```python
from build123d import *

# Parameters (mm, degrees)
SKETCH_1_W                       = 34.251173864
SKETCH_1_H                       = 50
EXTRUDE_1_DEPTH                  = 3
SKETCH_2_W                       = 3
SKETCH_2_H                       = 50
EXTRUDE_2_DEPTH                  = 50
SKETCH_3_R                       = 1
CUT_EXTRUDE_1_DEPTH              = 50
PATTERN_LINEAR_1_COUNT           = 3
PATTERN_LINEAR_1_PITCH           = 8
PATTERN_LINEAR_2_COUNT           = 3
PATTERN_LINEAR_2_PITCH           = 8
PATTERN_LINEAR_2_COPY_1_SKETCH_R = 1
PATTERN_LINEAR_2_COPY_1_DEPTH    = 50
PATTERN_LINEAR_2_COPY_2_SKETCH_R = 1
PATTERN_LINEAR_2_COPY_2_DEPTH    = 50
PATTERN_LINEAR_2_COPY_3_SKETCH_R = 1
PATTERN_LINEAR_2_COPY_3_DEPTH    = 50
PATTERN_LINEAR_2_COPY_4_SKETCH_R = 1
PATTERN_LINEAR_2_COPY_4_DEPTH    = 50


with BuildPart() as part:
    # 草图1 → 凸台-拉伸1 (new body)
    with BuildSketch(Plane(origin=(0, 0, 0), x_dir=(1, 0, 0), z_dir=(0, 1, 0))):
        with Locations((17.125586932, 0)):
            Rectangle(SKETCH_1_W, SKETCH_1_H)
    extrude(amount=EXTRUDE_1_DEPTH)

    # 草图2 → 凸台-拉伸2 (add)
    with BuildSketch(Plane(origin=(0, 3, 0), x_dir=(1, 0, 0), z_dir=(0, 1, 0))):
        with Locations((1.5, 0)):
            Rectangle(SKETCH_2_W, SKETCH_2_H)
    extrude(amount=EXTRUDE_2_DEPTH)

    # 草图3 → 切除-拉伸1 (cut)
    with BuildSketch(Plane.ZY):
        with Locations((-8, 39.156069013)):
            Circle(SKETCH_3_R)
    cut_extrude_1 = extrude(amount=-CUT_EXTRUDE_1_DEPTH, mode=Mode.SUBTRACT)

    # 阵列(线性)1: 切除-拉伸1 ×3
    with Locations(*[(0, 0, i * PATTERN_LINEAR_1_PITCH) for i in range(1, PATTERN_LINEAR_1_COUNT)]):
        add(cut_extrude_1, mode=Mode.SUBTRACT)

    # 阵列(线性)2: 切除-拉伸1 ×3
    with Locations(*[(0, -i * PATTERN_LINEAR_2_PITCH, 0) for i in range(1, PATTERN_LINEAR_2_COUNT)]):
        add(cut_extrude_1, mode=Mode.SUBTRACT)

    # 阵列(线性)2 copy 1 sketch → 阵列(线性)2 copy 1 (cut)
    with BuildSketch(Plane(origin=(0, -8, 8), x_dir=(0, 0, 1), z_dir=(-1, 0, 0))):
        with Locations((-8, 39.156069013)):
            Circle(PATTERN_LINEAR_2_COPY_1_SKETCH_R)
    extrude(amount=-PATTERN_LINEAR_2_COPY_1_DEPTH, mode=Mode.SUBTRACT)

    # 阵列(线性)2 copy 2 sketch → 阵列(线性)2 copy 2 (cut)
    with BuildSketch(Plane(origin=(0, -16, 8), x_dir=(0, 0, 1), z_dir=(-1, 0, 0))):
        with Locations((-8, 39.156069013)):
            Circle(PATTERN_LINEAR_2_COPY_2_SKETCH_R)
    extrude(amount=-PATTERN_LINEAR_2_COPY_2_DEPTH, mode=Mode.SUBTRACT)

    # 阵列(线性)2 copy 3 sketch → 阵列(线性)2 copy 3 (cut)
    with BuildSketch(Plane(origin=(0, -8, 16), x_dir=(0, 0, 1), z_dir=(-1, 0, 0))):
        with Locations((-8, 39.156069013)):
            Circle(PATTERN_LINEAR_2_COPY_3_SKETCH_R)
    extrude(amount=-PATTERN_LINEAR_2_COPY_3_DEPTH, mode=Mode.SUBTRACT)

    # 阵列(线性)2 copy 4 sketch → 阵列(线性)2 copy 4 (cut)
    with BuildSketch(Plane(origin=(0, -16, 16), x_dir=(0, 0, 1), z_dir=(-1, 0, 0))):
        with Locations((-8, 39.156069013)):
            Circle(PATTERN_LINEAR_2_COPY_4_SKETCH_R)
    extrude(amount=-PATTERN_LINEAR_2_COPY_4_DEPTH, mode=Mode.SUBTRACT)


solid = part.part
```
CAD build for the part. Positions are in the model's coordinates, mm. A direction names the side the tool comes from. Coordinates: 2 decimals unless noted, no trailing zeros. Order: outer loops, then holes, each group sorted by start corner. A loop starts at its lowest first (then second) coordinate and runs counter-clockwise, first axis right, second up. Notation, with made-up numbers: (55.5, 48.5) - (93.5, 48.5) arc R29 ccw to (93.5, 79.5) - close; hole circle Ø5 at (32.5, 2). An arc over 180 degrees is marked (long way). Use a Markdown table: item, result. Add a question column.
(1) Drill centre lines: line 1 along Y through (x, z) = (1.65, -8); line 2 along Y through (x, z) = (26, -3). Where is each one in solid material? Low to high. Write a range as [from, to].
(2) Saw through at B-B (z = 21). Give the cut face in (x, y).
(3) Pull direction Z, two halves, no side cores. Call faces 1 (the face through (2, 15, 25)), 2 (the face through (18, 3, 0)), 3 (the face through (1.48, 31.83, 7.26)): +Z half, -Z half, draft (parallel to the pull), parting line (faces both ways), or undercut.
(4) Saw through at A-A (z = 8). Give the cut face in (x, y), then the cut area to 3 significant figures.
(5) Flat gauge pins, fed straight in: pin 1 (2.5 mm diameter, centred on y = 23.16, z = -8, fed in from +X); pin 2 (2 mm diameter, centred on x = 6.5, z = 3.5, fed in from +Y). Where does each tip first touch, or does it go through?
(6) Which spindle directions (+Z, -Z, +X, -X, +Y, -Y) get a long thin tool onto all of the face, cutting with end or side? Do faces 4 (the face through (3, 28, 0)), 5 (the face through (1.479, 40.148, -8.13)). Say none if no direction does.
(7) Saw through at C-C (y = 49). Give the cut face in (x, z), then the cut area to 3 significant figures.
Solved:
| question | item | result |
|---|---|---|
| 1 | line 1 | y = [0, 22.16], [24.16, 30.16], [32.16, 38.16], [40.16, 53] |
| 1 | line 2 | y = [0, 3] |
| 2 | outline | (0, 0) - (34.25, 0) - (34.25, 3) - (3, 3) - (3, 53) - (0, 53) - close |
| 3 | face 1 | +Z half |
| 3 | face 2 | draft |
| 3 | face 3 | undercut |
| 4 | outline | (0, 0) - (34.25, 0) - (34.25, 3) - (3, 3) - (3, 22.16) - (0, 22.16) - close; (0, 24.16) - (3, 24.16) - (3, 30.16) - (0, 30.16) - close; (0, 32.16) - (3, 32.16) - (3, 38.16) - (0, 38.16) - close; (0, 40.16) - (3, 40.16) - (3, 53) - (0, 53) - close |
| 4 | area | 235 mm² |
| 5 | pin 1 | stops at x = 3 |
| 5 | pin 2 | stops at y = 3 |
| 6 | face 4 | +Z, -Z, +X, +Y |
| 6 | face 5 | +X, -X |
| 7 | outline | (0, -25) - (3, -25) - (3, 25) - (0, 25) - close |
| 7 | area | 150 mm² |
